from build123d import *

# Parameters (mm, degrees)
RESSALTO_EXTRUS_O1_DEPTH = 6
ESBO_O2_W                = 2.2
ESBO_O2_H                = 20
ESBO_O2_W_2              = 20
ESBO_O2_H_2              = 2.2
CORTE_EXTRUS_O1_DEPTH    = 6


with BuildPart() as part:
    # Esboço1 → Ressalto-extrusão1 (new body)
    with BuildSketch(Plane.XY):
        Polygon((150.105265805, 0), (179.905265805, 0), (179.905265805, 6), (202.8, 6), (202.8, 18.6), (209, 18.6), (209, 48.4), (202.8, 48.4), (202.8, 138.6), (209, 138.6), (209, 168.4), (202.8, 168.4), (202.8, 181), (179.905265805, 181), (179.905265805, 187), (150.105265805, 187), (150.105265805, 181), (57.605265805, 181), (57.605265805, 187), (27.805265805, 187), (27.805265805, 181), (0, 181), (0, 6), (27.805265805, 6), (27.805265805, 0), (57.605265805, 0), (57.605265805, 6), (150.105265805, 6), align=None)
    extrude(amount=RESSALTO_EXTRUS_O1_DEPTH)

    # Esboço2 → Corte-extrusão1 (cut)
    with BuildSketch(Plane.XY.offset(6)):
        with Locations((103.857898708, 171)):
            Rectangle(ESBO_O2_W, ESBO_O2_H)
        with Locations((192.8, 93.5)):
            Rectangle(ESBO_O2_W_2, ESBO_O2_H_2)
        with Locations((103.857898708, 16)):
            Rectangle(ESBO_O2_W, ESBO_O2_H)
    extrude(amount=-CORTE_EXTRUS_O1_DEPTH, mode=Mode.SUBTRACT)


solid = part.part
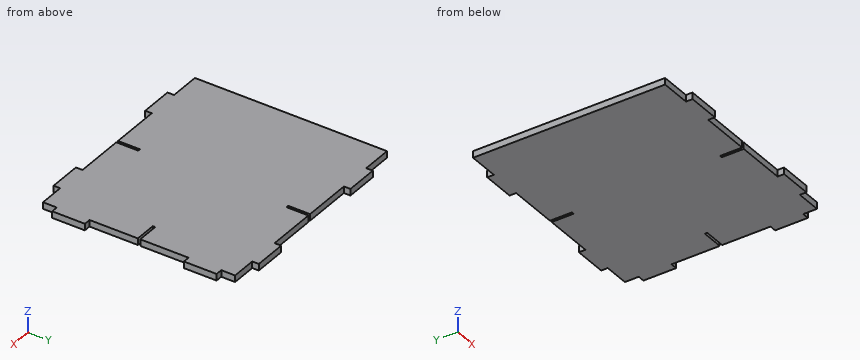
Geometry check sheet. Reference: the model listing, model coordinates, mm. Give positions to 0.01 mm unless a question says otherwise; leave off trailing zeros. Write each loop counter-clockwise with the first axis right and the second up, starting at its lowest first coordinate (ties: lowest second). Pieces come first, ordered by that corner, then holes. Notation, with made-up numbers: M 66,60 L 72,60 A22 cw 72,78 Z; hole C 69.5,81.5 d2. An arc over 180 degrees is marked long. Answer as CSV lines item,"result". Start each with the question number.
Q1. Section check B-B, the plane x = 63. Record the cut outline in (y, z).
Q2. Section check C-C, the plane y = 74. Record the cut outline in (x, z).
Q3. Material ranges on L1, parallel to X at y = 22, z = 1.85; L2, parallel to Y at x = 85.5, z = 0.3; L3, parallel to X at y = 99, z = 0.9, recorded low to high.
Q4. Go/stop test with flat-tipped pins: pin 1 (1.8 mm diameter, centred on y = 175.5, z = 2.5, fed in from +X); pin 2 (1.8 mm diameter, centred on x = 103.5, z = 3, fed in from +Y); pin 3 (1.8 mm diameter, centred on y = 184.5, z = 4, fed in from -X). Record where each tip stops, or that it passes through.
Q5. Section check A-A, the plane y = 15.5. Record the cut outline in (x, z).
Geometry says:
1,outline,"M 6,0 L 181,0 L 181,6 L 6,6 Z"
2,outline,"M 0,0 L 202.8,0 L 202.8,6 L 0,6 Z"
3,L1,"0 to 102.76, 104.96 to 209"
3,L2,"6 to 181"
3,L3,"0 to 202.8"
4,pin 1,"x = 202.8"
4,pin 2,"y = 181"
4,pin 3,"x = 27.81"
5,outline,"M 0,0 L 102.76,0 L 102.76,6 L 0,6 Z; M 104.96,0 L 202.8,0 L 202.8,6 L 104.96,6 Z"
